Autodesk Inventor part; units mm, degrees
ref_plane "YZ Plane" through (0, 0, 0) normal (1, 0, 0) x (0, 1, 0)
ref_plane "XZ Plane" through (0, 0, 0) normal (0, 1, 0) x (-1, 0, 0)
ref_plane "XY Plane" through (0, 0, 0) normal (0, 0, 1) x (1, 0, 0)
sketch "Sketch1" plane through (0, 0, 0) normal (1, 0, 0) x (0, 1, 0)
  line L0 (0, 0) -> (25.4, 0)
  line L1 (25.4, 0) -> (25.4, 3.175)
  line L2 (25.4, 3.175) -> (3.175, 3.175)
  line L3 (3.175, 3.175) -> (3.175, 25.4)
  line L4 (3.175, 25.4) -> (0, 25.4)
  line L5 (0, 25.4) -> (0, 0)
  dimension "d0" = 25.4
  dimension "d1" = 25.4
  dimension "d2" = 3.175
  dimension "d3" = 3.175
extrude "Extrusion1" add sketch "Sketch1" along normal blind 25.4
sketch "Sketch2" plane through (0, 3.175, 3.175) normal (0, 0, 1) x (1, 0, 0)
  line L0 (25.4, -3.175) -> (25.4, 22.225)
  line L1 (0, 22.225) -> (25.4, 22.225)
  point P0 (0, -3.175)
  point P1 (12.7, 15.875)
  dimension "d6" = 12.7
  dimension "d7" = 6.35
hole "Hole1" at (12.7, 19.05, 3.175) direction (0, 0, -1) diameter 6.7469 end through all
sketch "Sketch3" plane through (0, 3.175, 25.4) normal (0, 1, 0) x (1, 0, 0)
  line L0 (0, 25.4) -> (25.4, 25.4)
  line L1 (25.4, 22.225) -> (25.4, 0)
  point P0 (12.7, 12.7)
  dimension "d15" = 12.7
  dimension "d16" = 12.7
hole "Hole2" at (12.7, 3.175, 12.7) direction (0, -1, 0) diameter 12.7 end through all
properties part number "15102898-16-P-0313"
The model under review builds one solid part; all positions refer to its coordinate system, in mm. A direction names the side the tool comes from. Round coordinates to 2 decimals unless told otherwise and drop trailing zeros. Loops run counter-clockwise (first coordinate to the right, second up) from the corner with the lowest first, then second, coordinate; pieces in that order, holes last. Notation, with made-up numbers: (-31.75, 15.25) -> (-22.75, 15.25) arc R18 cw to (-22.75, 35.25) -> close; hole circle Ø6 at (67, 5.25). An arc over 180 degrees is marked (long way). Answer as a JSON object with one key per item and string values. Group by question number.
1) We need section D-D on y = 13.5. Write out the cut boundary in (x, z) (3 decimals).
2) For line 1 (Y direction, x = 12.7, z = 0.75); line 2 (Z direction, x = 12.7, y = 0.95), list the stretches that pass through material, from the lowest coordinate up. Write a range as [from, to].
3) We need section A-A on z = 12.7. Write out the cut boundary in (x, y) (3 decimals).
4) For pin 1 Ø2 at (x, y) = (15, 20.5) entering from +Z (3 decimals), flat-tipped, find the tip position at first contact; note if it passes through.
5) For faces 1 (the face through (16.56, 1.57, 7.66)), 2 (the face through (15, 3.175, 19)), list the 3-axis set-ups (+Z, -Z, +X, -X, +Y, -Y) from which the entire face can be reached by the end or side of a thin tool; tool diameter is ignored.
6) We need section C-C on y = 19.05. Write out the cut boundary in (x, z) (3 decimals), then the cut area to 3 significant figures.
7) Mouldability with a two-part tool opening along X and no side actions: class faces 3 (the face through (13, 14, 3.175)), 4 (the face through (25.4, 7, 2)), 5 (the face through (9.355, 19.489, 1.565)) as released by +X, released by -X, zero draft, split by the parting line, or undercut.
8) We need section B-B on x = 12.7. Write out the cut boundary in (y, z) (3 decimals).
Result set:
{
 "1": {"outline": "(0, 0) -> (25.4, 0) -> (25.4, 3.175) -> (0, 3.175) -> close"},
 "2": {"line 1": "[0, 15.68], [22.42, 25.4]", "line 2": "[0, 6.35], [19.05, 25.4]"},
 "3": {"outline": "(0, 0) -> (6.35, 0) -> (6.35, 3.175) -> (0, 3.175) -> close; (19.05, 0) -> (25.4, 0) -> (25.4, 3.175) -> (19.05, 3.175) -> close"},
 "4": {"pin 1": "z = 3.175"},
 "5": {"face 1": "+Y, -Y", "face 2": "+Z, +X, -X, +Y"},
 "6": {"outline": "(0, 0) -> (9.327, 0) -> (9.327, 3.175) -> (0, 3.175) -> close; (16.073, 0) -> (25.4, 0) -> (25.4, 3.175) -> (16.073, 3.175) -> close", "area": "59.2 mm²"},
 "7": {"face 3": "zero draft", "face 4": "released by +X", "face 5": "undercut"},
 "8": {"outline": "(0, 0) -> (15.677, 0) -> (15.677, 3.175) -> (3.175, 3.175) -> (3.175, 6.35) -> (0, 6.35) -> close; (0, 19.05) -> (3.175, 19.05) -> (3.175, 25.4) -> (0, 25.4) -> close; (22.423, 0) -> (25.4, 0) -> (25.4, 3.175) -> (22.423, 3.175) -> close"}
}
